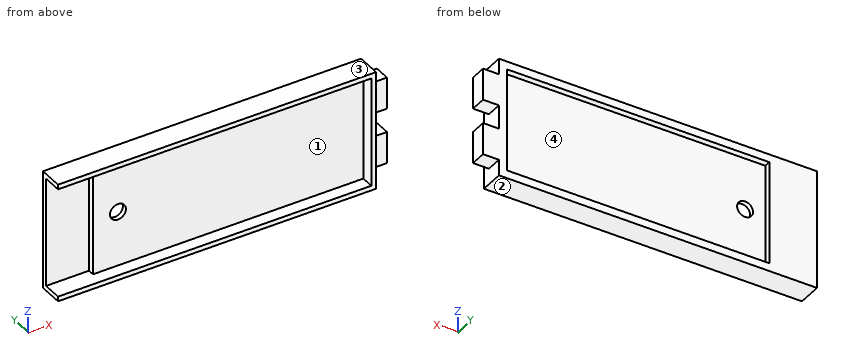
from build123d import *

# Parameters (mm, degrees)
SKETCH1_W           = 200
SKETCH1_H           = 75
BOSS_EXTRUDE1_DEPTH = 15
SKETCH9_W           = 165
SKETCH9_H           = 65
CUT_EXTRUDE5_DEPTH  = 4
SHELL3_START        = -34.5
SHELL3_DEPTH        = 69
SKETCH14_W          = 20
SKETCH14_H          = 10
BOSS_EXTRUDE5_DEPTH = 10
SKETCH15_R          = 5
CUT_EXTRUDE7_DEPTH  = 156.007257895


# Read off the part's stored shape, not the designer's step: Shell3
with BuildPart() as part:
    # Sketch1 → Boss-Extrude1 (new body)
    with BuildSketch(Plane(origin=(0, 0, 0), x_dir=(1, 0, 0), z_dir=(0, 1, 0))):
        with Locations((40, 0)):
            Rectangle(SKETCH1_W, SKETCH1_H)
    extrude(amount=BOSS_EXTRUDE1_DEPTH)

    # Sketch9 → Cut-Extrude5 (cut)
    with BuildSketch(Plane(origin=(0, 15, 0), x_dir=(1, 0, 0), z_dir=(0, 1, 0))):
        with Locations((52.5, 0)):
            Rectangle(SKETCH9_W, SKETCH9_H)
    extrude(amount=-CUT_EXTRUDE5_DEPTH, mode=Mode.SUBTRACT)

    # Shell3 outline → Shell3 (cut)
    with BuildSketch(Plane.XY.offset(SHELL3_START)):
        Polygon((137, 0), (137, 8), (-33, 8), (-33, 12), (-60, 12), (-60, 0), align=None)
    extrude(amount=SHELL3_DEPTH, mode=Mode.SUBTRACT)

    # Sketch14 → Boss-Extrude5 (add)
    with BuildSketch(Plane(origin=(140, 0, 0), x_dir=(0, 0, -1), z_dir=(1, 0, 0))):
        with Locations((-17.5, 10)):
            Rectangle(SKETCH14_W, SKETCH14_H)
        with Locations((17.5, 10)):
            Rectangle(SKETCH14_W, SKETCH14_H)
    extrude(amount=BOSS_EXTRUDE5_DEPTH)

    # Sketch15 → Cut-Extrude7 (cut, through all)
    with BuildSketch(Plane(origin=(0, 11, 0), x_dir=(1, 0, 0), z_dir=(0, 1, 0))):
        with Locations(Location((-17.28231035, 0, 0), (0, 0, 270))):
            Circle(SKETCH15_R)
    extrude(amount=-CUT_EXTRUDE7_DEPTH, mode=Mode.SUBTRACT)


solid = part.part
Geometry: final body of the model. Coordinates: model frame, mm. Face numbers are marked on the shaded views. A direction names the side the tool comes from. Give positions to 0.01 mm unless a question says otherwise; leave off trailing zeros. Order: outer loops, then holes, each group sorted by start corner. A loop starts at its lowest first (then second) coordinate and runs counter-clockwise, first axis right, second up. Notation, with made-up numbers: (14, -6) -> (71, -6) arc R16 cw to (71, 13) -> close; hole circle Ø8 at (35, -4.5). An arc over 180 degrees is marked (long way). Put each result on its own line as item: value.
Q1. Draft query along X for the marked faces 3 and 4. Return one class per face: released by +X, released by -X, zero draft, split by the parting line, or undercut.
Here are the results:
face 3: zero draft
face 4: undercut
Q2. Reachability of the marked faces 1 and 2 from +Z, -Z, +X, -X, +Y, -Y: full face, straight path, thin tool, end or side. Return the list, or none.
Here are the results:
face 1: -X, -Y
face 2: -Z, +X, -X, +Y, -Y
Q3. Pin query (flat end, axial travel): pin 1 (5 mm diameter, centred on x = 145, y = 10, fed in from +Z); pin 2 (1 mm diameter, centred on x = 88.5, z = 25.5, fed in from +Y); pin 3 (3 mm diameter, centred on x = 147, z = 18, fed in from -Y). Return the tip coordinate at first contact, or that it passes through.
Here are the results:
pin 1: stops at z = 27.5
pin 2: stops at y = 11
pin 3: stops at y = 5
Q4. Section B-B, the plane x = 34.5. Return loops of the section in (y, z).
Here are the results:
outline: (0, -37.5) -> (15, -37.5) -> (15, -32.5) -> (11, -32.5) -> (11, 32.5) -> (15, 32.5) -> (15, 37.5) -> (0, 37.5) -> (0, 34.5) -> (8, 34.5) -> (8, -34.5) -> (0, -34.5) -> close
Q5. Material intervals for L1, parallel to Z at x = -20, y = 5.5; L2, parallel to X at y = 10.35, z = 0; L3, parallel to Z at x = 46, y = 14.5, sorted ascending.
Here are the results:
L1: z = -37.5 to -34.5, 34.5 to 37.5
L2: x = -33 to -22.28, -12.28 to 140
L3: z = -37.5 to -32.5, 32.5 to 37.5
Q6. Section C-C, the plane z = -20. Return loops of the section in (x, y), then the cut area to 3 significant figures.
Here are the results:
outline: (-60, 12) -> (-33, 12) -> (-33, 8) -> (137, 8) -> (137, 0) -> (140, 0) -> (140, 5) -> (150, 5) -> (150, 15) -> (135, 15) -> (135, 11) -> (-30, 11) -> (-30, 15) -> (-60, 15) -> close
area: 756 mm^2
Q7. Section A-A, the plane z = 0. Return loops of the section in (x, y), then the cut area to 3 significant figures.
Here are the results:
outline: (-60, 12) -> (-33, 12) -> (-33, 8) -> (-22.28, 8) -> (-22.28, 11) -> (-30, 11) -> (-30, 15) -> (-60, 15) -> close; (-12.28, 8) -> (137, 8) -> (137, 0) -> (140, 0) -> (140, 15) -> (135, 15) -> (135, 11) -> (-12.28, 11) -> close
area: 626 mm^2
